Read the model definition and answer for the solid it produces. Units are mm, in the model's axes. A direction names the side the tool comes from. Round coordinates to 2 decimals unless told otherwise and drop trailing zeros. Write each loop counter-clockwise with the first axis right and the second up, starting at its lowest first coordinate (ties: lowest second). Pieces come first, ordered by that corner, then holes. Notation, with made-up numbers: M 46.25,23 L 83.25,23 A19 ccw 83.25,57 Z; hole C 33.25,19 d1. An arc over 180 degrees is marked long. Use one line per item in the form item = value. Start each with the question number.
```python
from build123d import *

# Parameters (mm, degrees)
SKETCH_1_W          = 13
SKETCH_1_H          = 6.8
EXTRUDE_1_DEPTH     = 14
SKETCH_3_W          = 13
SKETCH_3_H          = 8.8
CUT_EXTRUDE_1_DEPTH = 1
EXTRUDE_2_DEPTH     = 0.2
SKETCH_6_W          = 12.6
SKETCH_6_H          = 5.4
CUT_EXTRUDE_2_DEPTH = 9
SKETCH_7_W          = 10
SKETCH_7_H          = 2
EXTRUDE_3_DEPTH     = 8.5
CHAMFER_1_SIZE      = 0.5


with BuildPart() as part:
    # 草图1 → 拉伸1 (new body)
    with BuildSketch(Plane.XY):
        Rectangle(SKETCH_1_W, SKETCH_1_H)
    extrude(amount=EXTRUDE_1_DEPTH)

    # 草图3 → 切除-拉伸1 (cut)
    with BuildSketch(Plane(origin=(0, 3.4, 0), x_dir=(-1, 0, 0), z_dir=(0, 1, 0))):
        with Locations((0, 4.6)):
            Rectangle(SKETCH_3_W, SKETCH_3_H)
    extrude(amount=-CUT_EXTRUDE_1_DEPTH, mode=Mode.SUBTRACT)

    # 草图4 → 拉伸2 (add)
    with BuildSketch(Plane(origin=(0, 0, 0), x_dir=(-1, 0, 0), z_dir=(0, 0, -1))):
        Polygon((-7.5, 2.4), (7.5, 2.4), (7.5, -3.4), (6.5, -3.4), (6.5, -4.4), (-6.5, -4.4), (-6.5, -3.4), (-7.5, -3.400976197), align=None)
    extrude(amount=-EXTRUDE_2_DEPTH)

    # 草图6 → 切除-拉伸2 (cut)
    with BuildSketch(Plane(origin=(0, 0, 0), x_dir=(-1, 0, 0), z_dir=(0, 0, -1))):
        with Locations((0, -0.5)):
            Rectangle(SKETCH_6_W, SKETCH_6_H)
    extrude(amount=-CUT_EXTRUDE_2_DEPTH, mode=Mode.SUBTRACT)

    # 草图7 → 拉伸3 (add)
    with BuildSketch(Plane(origin=(0, 0, 9), x_dir=(-1, 0, 0), z_dir=(0, 0, -1))):
        with Locations((0, -1.2)):
            Rectangle(SKETCH_7_W, SKETCH_7_H)
    extrude(amount=EXTRUDE_3_DEPTH)

    # 倒角1
    chamfer_1_edges = [part.edges().sort_by_distance(p)[0] for p in [
        (0, -0.2, 0.5),
        (-5, -1.2, 0.5),
        (0, -2.2, 0.5),
        (5, -1.2, 0.5),
    ]]
    chamfer(chamfer_1_edges, length=CHAMFER_1_SIZE)


solid = part.part
```
Q1. Find section A-A on z = 7.75. Write down the section's boundary in (x, y).
Q2. Straight lines are drawn through the part: line 1 (X direction, y = -0.25, z = 3.5); line 2 (Y direction, x = 2.5, z = 3.75); line 3 (Z direction, x = -5, y = 2.5). For each, find the intervals that lie inside material, in ascending order. Write a range as [from, to].
Q3. Find section D-D on z = 10.75. Write down the section's boundary in (x, y).
Q4. Find section C-C on y = -1.25. Write down the section's boundary in (x, z).
Q5. For a pull along Y with two mould halves and no side action, classify faces 5 (the face through (0, 0, 9)), 6 (the face through (0, -3.4, 7)), 7 (the face through (7, 0, 0.2)) as +Y half, -Y half, draft (parallel to the pull), parting line (faces both ways), or undercut.
Q6. A tool of negligible diameter and unlimited length cuts with its end or side. For faces 1 (the face through (-5, -1, 5)), 2 (the face through (-7, 0, 0.2)), 3 (the face through (0, 3, 9)), 4 (the face through (6.5, 0, 7)), from which of +Z, -Z, +X, -X, +Y, -Y can it reach the whole face along a straight path? Write none if from no direction.
Q7. Find section B-B on x = 5.5. Write down the section's boundary in (y, z).
Q8. Each of these flat-tipped pins is pushed along its axis until it touches: pin 1 Ø1.5 at (y, z) = (2.5, 3.5) entering from +X; pin 2 Ø4 at (x, z) = (-2, 4) entering from -Y; pin 3 Ø2 at (y, z) = (-2.5, 7) entering from -X. Where does it stop, or does it pass through?
Response:
q1.outline = M -6.5,-3.4 L 6.5,-3.4 L 6.5,2.4 L -6.5,2.4 Z; M -5,-2.2 L 5,-2.2 L 5,-0.2 L -5,-0.2 Z; hole M -6.3,-3.2 L 6.3,-3.2 L 6.3,2.2 L -6.3,2.2 Z
q2.line_1 = [-6.5, -6.3], [-5, 5], [6.3, 6.5]
q2.line_2 = [-3.4, -3.2], [-2.2, -0.2], [2.2, 2.4]
q2.line_3 = [0, 0.2], [9, 14]
q3.outline = M -6.5,-3.4 L 6.5,-3.4 L 6.5,3.4 L -6.5,3.4 Z
q4.outline = M -7.5,0 L -6.3,0 L -6.3,9 L -5,9 L -5,1 L -4.5,0.5 L 4.5,0.5 L 5,1 L 5,9 L 6.3,9 L 6.3,0 L 7.5,0 L 7.5,0.2 L 6.5,0.2 L 6.5,14 L -6.5,14 L -6.5,0.2 L -7.5,0.2 Z
q5.face_5 = undercut
q5.face_6 = -Y half
q5.face_7 = draft
q6.face_1 = -Z
q6.face_2 = +Z, -X, +Y, -Y
q6.face_3 = +X, -X, +Y
q6.face_4 = +Z, +X, +Y, -Y
q7.outline = M -4.4,0 L -3.2,0 L -3.2,9 L 2.2,9 L 2.2,0 L 3.4,0 L 3.4,0.2 L 2.4,0.2 L 2.4,9 L 3.4,9 L 3.4,14 L -3.4,14 L -3.4,0.2 L -4.4,0.2 Z
q8.pin_1 = 6.5
q8.pin_2 = -3.4
q8.pin_3 = -6.5
